Check sheet for the modelled part. Datum: model origin and axes. Units: mm. A direction names the side the tool comes from. Round coordinates to 2 decimals unless told otherwise and drop trailing zeros. Write each loop counter-clockwise with the first axis right and the second up, starting at its lowest first coordinate (ties: lowest second). Pieces come first, ordered by that corner, then holes. Notation, with made-up numbers: (-29, -27.5) -> (6, -27.5) arc R18 cw to (6, -11.5) -> close; hole circle Ø5 at (-13.5, 16.25). An arc over 180 degrees is marked (long way). Write item = value, one per line.
from build123d import *

# Parameters (mm, degrees)
SKETCH_1_R          = 16
SKETCH_1_R_2        = 14.3
EXTRUDE_1_DEPTH     = 4
SKETCH_2_R          = 20
EXTRUDE_2_DEPTH     = 2
SKETCH_3_R          = 14.3
CUT_EXTRUDE_1_DEPTH = 2


with BuildPart() as part:
    # 草图1 → 凸台-拉伸1 (new body)
    with BuildSketch(Plane.XY):
        Circle(SKETCH_1_R)
        Circle(SKETCH_1_R_2, mode=Mode.SUBTRACT)
    extrude(amount=EXTRUDE_1_DEPTH)

    # 草图2 → 凸台-拉伸2 (add)
    with BuildSketch(Plane.XY.offset(4)):
        Circle(SKETCH_2_R)
    extrude(amount=EXTRUDE_2_DEPTH)

    # 草图3 → 切除-拉伸1 (cut)
    with BuildSketch(Plane(origin=(0, 0, 4), x_dir=(-1, 0, 0), z_dir=(0, 0, -1))):
        Circle(SKETCH_3_R)
    extrude(amount=-CUT_EXTRUDE_1_DEPTH, mode=Mode.SUBTRACT)


solid = part.part
(1) Material ranges on L1, parallel to Y at x = 0, z = 1.05; L2, parallel to Y at x = 0, z = 5.65; L3, parallel to X at y = 9, z = 3.45, recorded low to high. Write a range as [from, to].
Worked answers:
L1 = [-16, -14.3], [14.3, 16]
L2 = [-20, -14.3], [14.3, 20]
L3 = [-13.23, -11.11], [11.11, 13.23]
(2) Sectioned sample at D-D on z = 4.7. Enter the section's corners in (x, y).
Worked answers:
outline = circle Ø40 at (0, 0); hole circle Ø28.6 at (0, 0)
(3) Access from +Z, -Z, +X, -X, +Y, -Y to the whole of each face (thin tool, end or side, straight path). Record for faces 1 (the cylindrical face through (-3.47, -15.62, 1.97)), 2 (the flat face through (-5, 14, 6)).
Worked answers:
face_1 = -Z
face_2 = +Z, +X, -X, +Y, -Y
(4) Sectioned sample at C-C on z = 1.45. Enter the section's corners in (x, y), then the cut area to 3 significant figures.
Worked answers:
outline = circle Ø32 at (0, 0); hole circle Ø28.6 at (0, 0)
area = 162 mm²
(5) Go/stop test with flat-tipped pins: P1, Ø6, axis at x = -13.5, y = -2, coming from the +Z side; P2, Ø12, axis at x = -3.5, y = 1.5, coming from the -Z side; P3, Ø2, axis at y = 5, z = 1.5, coming from the +X side; P4, Ø1, axis at x = 15.5, y = -11.5, coming from the -Z side. Record where each tip stops, or that it passes through.
Worked answers:
P1 = 6
P2 = through
P3 = 15.49
P4 = 4
(6) Sectioned sample at A-A on y = 0. Enter the section's corners in (x, z).
Worked answers:
outline = (-20, 4) -> (-16, 4) -> (-16, 0) -> (-14.3, 0) -> (-14.3, 6) -> (-20, 6) -> close; (14.3, 0) -> (16, 0) -> (16, 4) -> (20, 4) -> (20, 6) -> (14.3, 6) -> close
